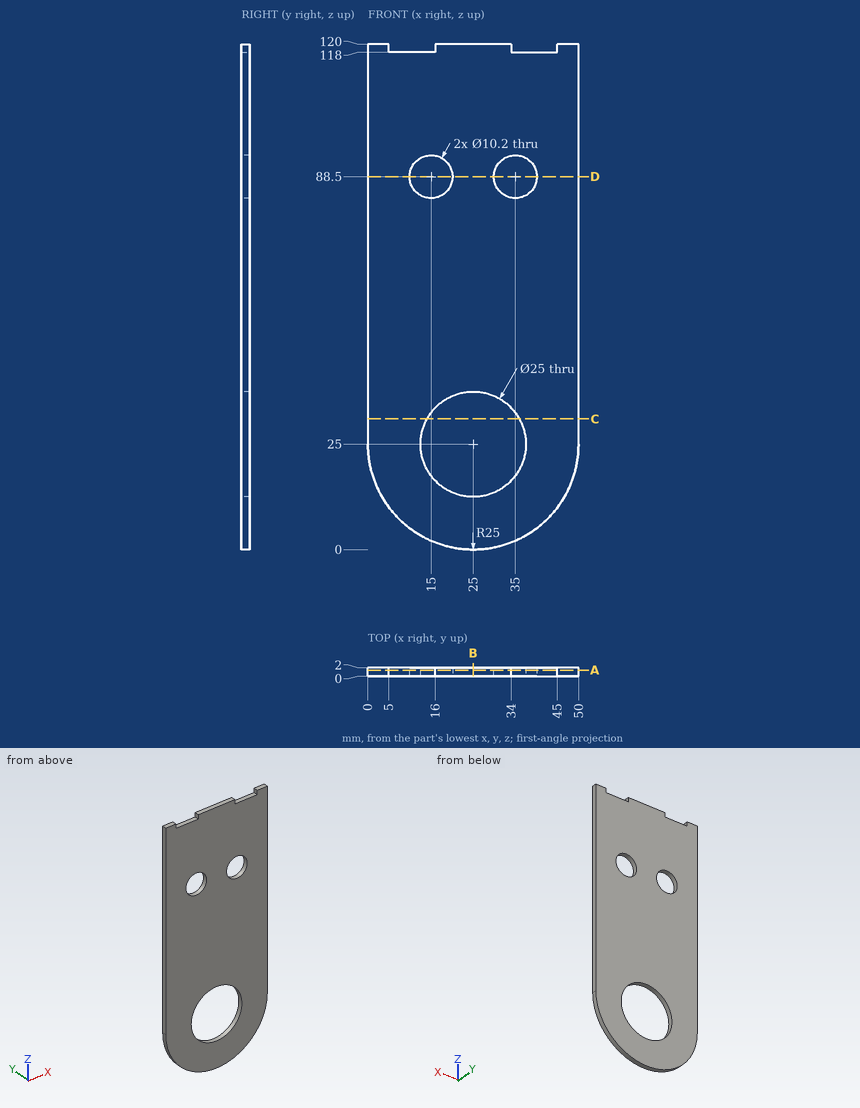
Design review of the part shown in the three views and the two pictorial views. Dimensions are in mm from the part's minimum x, y and z. Round coordinates to 2 decimals unless told otherwise and drop trailing zeros. Write each loop counter-clockwise with the first axis right and the second up, starting at its lowest first coordinate (ties: lowest second). Pieces come first, ordered by that corner, then holes. Notation, with made-up numbers: (-38.75, -27) -> (10.25, -27) arc R24 ccw to (10.25, -7) -> close; hole circle Ø6 at (67, 2). An arc over 180 degrees is marked (long way). Answer as a JSON object with one key per item and string values.
1. We need section A-A on y = 1.4. State the section outline as (x, z) points.
Results found:
{"outline": "(0, 25) arc R25 ccw to (50, 25) -> (50, 120) -> (45, 120) -> (45, 118) -> (34, 118) -> (34, 120) -> (16, 120) -> (16, 118) -> (5, 118) -> (5, 120) -> (0, 120) -> close; hole circle Ø10.2 at (15, 88.5); hole circle Ø25 at (25, 25); hole circle Ø10.2 at (35, 88.5)"}
2. We need section D-D on z = 88.5. State the section outline as (x, y) points.
Results found:
{"outline": "(0, 0) -> (9.9, 0) -> (9.9, 2) -> (0, 2) -> close; (20.1, 0) -> (29.9, 0) -> (29.9, 2) -> (20.1, 2) -> close; (40.1, 0) -> (50, 0) -> (50, 2) -> (40.1, 2) -> close"}
3. To check wall thickness, follow line 1 along Z through (x, y) = (33.5, 1); line 2 along Z through (x, y) = (25, 1.35); line 3 along X through (y, z) = (0.6, 90). State the ranges of each line that lie inside material, in increasing order.
Results found:
{"line 1": "z = 1.49 to 15.83, 34.17 to 83.63, 93.37 to 120", "line 2": "z = 0 to 12.5, 37.5 to 120", "line 3": "x = 0 to 10.13, 19.87 to 30.13, 39.87 to 50"}
4. We need section B-B on x = 25. State the section outline as (y, z) points, and give its area (3 significant figures).
Results found:
{"outline": "(0, 0) -> (2, 0) -> (2, 12.5) -> (0, 12.5) -> close; (0, 37.5) -> (2, 37.5) -> (2, 120) -> (0, 120) -> close", "area": "190 mm^2"}
5. We need section C-C on z = 31. State the section outline as (x, y) points.
Results found:
{"outline": "(0, 0) -> (14.03, 0) -> (14.03, 2) -> (0, 2) -> close; (35.97, 0) -> (50, 0) -> (50, 2) -> (35.97, 2) -> close"}
6. Clearance check with flat-ended pins moving along their axes: pin 1 (9 mm diameter, centred on x = 15, z = 88.5, fed in from -Y); pin 2 (1 mm diameter, centred on x = 12.5, y = 1, fed in from +Z). State where each tip first meets the part, or that it passes through.
Results found:
{"pin 1": "passes through", "pin 2": "stops at z = 118"}
